CAD build for the part. Positions are in the model's coordinates, mm. A direction names the side the tool comes from. Give positions to 0.01 mm unless a question says otherwise; leave off trailing zeros. Order: outer loops, then holes, each group sorted by start corner. A loop starts at its lowest first (then second) coordinate and runs counter-clockwise, first axis right, second up. Notation, with made-up numbers: (-36, 24.5) -> (-27, 24.5) arc R12 cw to (-27, 42.5) -> close; hole circle Ø8 at (66, -2.75). An arc over 180 degrees is marked (long way). Answer as CSV lines item,"result".
```python
from build123d import *

# Parameters (mm, degrees)
F0_W          = 3.81
F0_H          = 25.4
F1_DEPTH      = 7.62
F2_DEPTH      = 25.4
F2_DEPTH_BACK = 7.62
F4_DEPTH      = 30.48
F6_DEPTH      = 15.24
F6_FACE_W     = 12.7
F6_FACE_H     = 15.24
F7_DEPTH      = 38.1
F8_R          = 3.81
F9_DEPTH      = 25.4


with BuildPart() as f1:
    # F0 (on Front) → F1 (new body)
    with BuildSketch(Plane.XZ):
        Polygon((-25.266106, 34.727762), (-55.746106, 34.727762), (-55.746106, 9.327762), (-51.936106, 9.327762), (-51.936106, -16.072238), (-55.746106, -16.072238), (-55.746106, -41.472238), (-25.266106, -41.472238), (-25.266106, -16.072238), (-29.076106, -16.072238), (-29.076106, 9.327762), (-25.266106, 9.327762), align=None)
        with Locations((-53.841106, -3.372238)):
            Rectangle(F0_W, F0_H)
        with Locations((-27.171106, -3.372238)):
            Rectangle(F0_W, F0_H)
    extrude(amount=F1_DEPTH)

    # F0 (on Front) → F2 (join, two sides)
    with BuildSketch(Plane.XZ) as f2_sk:
        with Locations((-53.841106, -3.372238)):
            Rectangle(F0_W, F0_H)
        with Locations((-27.171106, -3.372238)):
            Rectangle(F0_W, F0_H)
    extrude(amount=-F2_DEPTH)
    extrude(f2_sk.sketch, amount=-F2_DEPTH_BACK)

    # F3 (on face) → F4 (join)
    with BuildSketch(Plane.YZ.offset(-25.266106)):
        with BuildLine():
            Line((-7.62, 34.727762), (0, 34.727762))
            Line((0, 34.727762), (0, 60.127762))
            Line((0, 60.127762), (-20.32, 60.127762))
            ThreePointArc((-20.32, 60.127762), (-16.700865, -4.418776), (0, -66.872238))
            Line((0, -66.872238), (0, -41.472238))
            Line((0, -41.472238), (-7.62, -41.472238))
            Line((-7.62, -41.472238), (-7.62, 34.727762))
        make_face()
    extrude(amount=-F4_DEPTH)

    # F5 (on face) → F6 (join)
    with BuildSketch(Plane.XY.offset(60.127762)):
        Polygon((-25.266106, 0), (-25.266106, -20.32), (1.674663, 6.620768), (14.374663, 19.320768), (1.674663, 19.320768), (-17.646106, 0), align=None)
        Polygon((-82.686874, 6.620768), (-55.746106, -20.32), (-55.746106, 0), (-63.366106, 0), (-82.686874, 19.320768), (-95.386874, 19.320768), align=None)
    extrude(amount=-F6_DEPTH)

    # F6_face (on face) → F7 (join)
    with BuildSketch(Plane(origin=(8.024663, 19.320768, 52.507762), x_dir=(-1, 0, 0), z_dir=(0, 1, 0))):
        Rectangle(F6_FACE_W, F6_FACE_H)
        with Locations((97.061537, 0)):
            Rectangle(F6_FACE_W, F6_FACE_H)
    extrude(amount=F7_DEPTH)

    # F8 (on face) → F9 (cut)
    with BuildSketch(Plane.XY.offset(60.127762)):
        with Locations((-89.036874, 49.800768)):
            Circle(F8_R)
        with Locations((-89.036874, 24.400768)):
            Circle(F8_R)
        with Locations((8.024663, 49.800768)):
            Circle(F8_R)
        with Locations((8.024663, 24.400768)):
            Circle(F8_R)
    extrude(amount=-F9_DEPTH, mode=Mode.SUBTRACT)


solid = f1.part
```
1) Band-saw the part on B-B, the plane x = -27. Write the cut outline in (y, z), then the cut area to 3 significant figures.
Data:
outline,"(-20.32, 60.13) arc R315.47 ccw to (0, -66.87) -> (0, -16.07) -> (25.4, -16.07) -> (25.4, 9.33) -> (0, 9.33) -> (0, 60.13) -> close"
area,"2,500 mm2"
2) Pin check, flat tips, straight feed: P1, Ø3, axis at x = -42.5, z = -39.5, coming from the -Y side; P2, Ø3, axis at x = -53, y = 14.5, coming from the +Z side; P3, Ø3, axis at x = -53, z = -5, coming from the +Y side; P4, Ø4.5, axis at x = -89.04, y = 24.4, coming from the -Z side. Stop position of each tip, or through.
Data:
P1,"stops at y = -9.43"
P2,"stops at z = 9.33"
P3,"stops at y = 25.4"
P4,"passes through"
3) Pull direction Y, two halves, no side cores. Call faces 5 (the cylindrical face through (7.53, 28.18, 52.61)), 6 (the flat face through (1.675, 38, 52)), 7 (the flat face through (-54, 25.4, -3)): pulls with the +Y half, pulls with the -Y half, needs draft (parallel to the pull), parting line crosses it, or undercut.
Data:
face 5,"undercut"
face 6,"needs draft"
face 7,"pulls with the +Y half"
4) Band-saw the part on A-A, the plane y = 38.5. Write the cut outline in (x, z).
Data:
outline,"(-95.39, 44.89) -> (-82.69, 44.89) -> (-82.69, 60.13) -> (-95.39, 60.13) -> close; (1.67, 44.89) -> (14.37, 44.89) -> (14.37, 60.13) -> (1.67, 60.13) -> close"
5) Which spindle directions (+Z, -Z, +X, -X, +Y, -Y) get a long thin tool onto all of the face, cutting with end or side? Do faces 1 (the flat face through (-27, 13, 9.328)), 2 (the flat face through (-51.936, 13, -4)), 3 (the flat face through (-54, 13, -16.072)), 4 (the flat face through (-83, 19, 44.888)). Say none if no direction does.
Data:
face 1,"+Z, +X, -X, +Y"
face 2,"+Z, -Z, +Y"
face 3,"-Z, +X, -X, +Y"
face 4,"-Z, -X, +Y, -Y"
6) Band-saw the part on C-C, the plane y = 13. Write the cut outline in (x, z).
Data:
outline,"(-89.07, 44.89) -> (-76.37, 44.89) -> (-76.37, 60.13) -> (-89.07, 60.13) -> close; (-55.75, -16.07) -> (-51.94, -16.07) -> (-51.94, 9.33) -> (-55.75, 9.33) -> close; (-29.08, -16.07) -> (-25.27, -16.07) -> (-25.27, 9.33) -> (-29.08, 9.33) -> close; (-4.65, 44.89) -> (8.05, 44.89) -> (8.05, 60.13) -> (-4.65, 60.13) -> close"
7) Band-saw the part on D-D, the plane z = 0.5. Write the cut outline in (x, y), then the cut area to 3 significant figures.
Data:
outline,"(-55.75, -17.45) -> (-25.27, -17.45) -> (-25.27, 25.4) -> (-29.08, 25.4) -> (-29.08, 0) -> (-51.94, 0) -> (-51.94, 25.4) -> (-55.75, 25.4) -> close"
area,"725 mm2"
8) Wall check: line 1 along X through (y, z) = (2.5, 7); line 2 along Z through (x, y) = (-87.5, 19); line 3 along Y through (x, z) = (-51, 43). Give the ranges that are in metal, low to high. Write a range as [from, to].
Data:
line 1,"x = [-55.75, -51.94], [-29.08, -25.27]"
line 2,"z = [44.89, 60.13]"
line 3,"y = [-20.65, 0]"
